Build history of the part. All positions in model axes, mm. A direction names the side the tool comes from. Coordinates: 2 decimals unless noted, no trailing zeros. Loops run counter-clockwise (first coordinate to the right, second up) from the corner with the lowest first, then second, coordinate; pieces in that order, holes last.
Item 1: Drill centre lines: line 1 along X through (y, z) = (11.5, 7); line 2 along Y through (x, z) = (11.5, 6.5); line 3 along X through (y, z) = (10, 8.5). Where is each one in solid material? Low to high.
Item 2: Flat gauge pins, fed straight in: pin 1 (1 mm diameter, centred on x = 0.5, y = 7.5, fed in from -Z); pin 2 (10 mm diameter, centred on x = -11, y = 5, fed in from +Z); pin 3 (4 mm diameter, centred on y = 10, z = -12, fed in from +X). Where does each tip first touch, or does it go through?
Item 3: Cut at C-C (z = 0). List the corners of the cut face in (x, y).
Item 4: Cut at D-D (x = 9.5). List the corners of the cut face in (y, z), and give its area (3 significant figures).
Item 5: Cut at B-B (x = 0). List the corners of the cut face in (y, z) (3 decimals).
Item 6: 3-axis set-ups, long thin cutter, end or side, ignore diameter. For faces 1 (the face through (0, -5, 0.75)), 2 (the face through (-11.03, 7.6, -2.19)), 3 (the face through (2, 15.5, 2)), 4 (the face through (0, -5, -1.5)): which of +Z, -Z, +X, -X, +Y, -Y reach the whole face in a straight line?
Item 7: Mould opens along X. For faces 5 (the face through (5.56, 7.6, 9.91)), 6 (the face through (9.498, 7.395, -12.876)), 7 (the face through (0, 24, -1.25)) say: released by +X, released by -X, zero draft, split by the parting line, or undercut.
from build123d import *

# Parameters (mm, degrees)
SKETCH_1_R               = 16
EXTRUDE_1_DEPTH          = 15
SKETCH_2_R               = 4
EXTRUDE_2_DEPTH          = 0.5
EXTRUDE_START            = 0.5
SKETCH_3_R               = 4
EXTRUDE_3_DEPTH          = 0.5
SKETCH_4_R               = 2.5
EXTRUDE_4_DEPTH          = 9.8
EXTRUDE_START_2          = 3
SKETCH_5_R               = 2.5
EXTRUDE_5_DEPTH          = 3
CUT_EXTRUDE_START        = -2.8
CUT_EXTRUDE_1_DEPTH      = 2.8
CUT_EXTRUDE_2_DEPTH      = 30.227555491
PATTERN_CIRCULAR_1_COUNT = 5
SKETCH_8_R               = 1.5
EXTRUDE_6_DEPTH          = 3
CHAMFER_1_SIZE           = 0.5
CUT_EXTRUDE_START_2      = -3
CUT_EXTRUDE_3_DEPTH      = 3


with BuildPart() as part:
    # 草图1 → 凸台-拉伸1 (new body)
    with BuildSketch(Plane(origin=(0, 0, 0), x_dir=(1, 0, 0), z_dir=(0, 1, 0))):
        with Locations(Location((0, 0, 0), (0, 0, 270))):
            Circle(SKETCH_1_R)
    extrude(amount=EXTRUDE_1_DEPTH)

    # 草图2 → 凸台-拉伸2 (add)
    with BuildSketch(Plane(origin=(0, 15, 0), x_dir=(1, 0, 0), z_dir=(0, 1, 0))):
        with Locations(Location((0, 0, 0), (0, 0, 270))):
            Circle(SKETCH_2_R)
    extrude(amount=EXTRUDE_2_DEPTH)

    # 草图3 → 凸台-拉伸3 (add)
    with BuildSketch(Plane.XZ.offset(EXTRUDE_START)):
        with Locations(Location((0, 0, 0), (0, 0, 90))):
            Circle(SKETCH_3_R)
    extrude(amount=-EXTRUDE_3_DEPTH)

    # 草图4 → 凸台-拉伸4 (add)
    with BuildSketch(Plane(origin=(0, 15.5, 0), x_dir=(1, 0, 0), z_dir=(0, 1, 0))):
        with Locations(Location((0, 0, 0), (0, 0, 270))):
            Circle(SKETCH_4_R)
    extrude(amount=EXTRUDE_4_DEPTH)

    # 草图5 → 凸台-拉伸5 (add)
    with BuildSketch(Plane.XZ.offset(0.5).offset(EXTRUDE_START_2)):
        with Locations(Location((0, 0, 0), (0, 0, 90))):
            Circle(SKETCH_5_R)
    extrude(amount=-EXTRUDE_5_DEPTH)

    # 草图6 → 切除-拉伸1 (cut)
    with BuildSketch(Plane(origin=(0, 25.3, 0), x_dir=(1, 0, 0), z_dir=(0, 1, 0)).offset(CUT_EXTRUDE_START)):
        with BuildLine():
            Line((-2.165063509, 1.25), (2.165063509, 1.25))
            ThreePointArc((2.165063509, 1.25), (0, 2.5), (-2.165063509, 1.25))
        make_face()
    extrude(amount=CUT_EXTRUDE_1_DEPTH, mode=Mode.SUBTRACT)

    # 草图7 → 切除-拉伸2 (cut, through all)
    with BuildSketch(Plane(origin=(0, 15, 0), x_dir=(1, 0, 0), z_dir=(0, 1, 0))):
        with BuildLine():
            Line((-1.325, 7), (-1.325, 19))
            Line((-1.325, 19), (1.325, 19))
            Line((1.325, 19), (1.325, 7))
            ThreePointArc((1.325, 7), (0, 5.675), (-1.325, 7))
        make_face()
    cut_extrude_2 = extrude(amount=-CUT_EXTRUDE_2_DEPTH, mode=Mode.SUBTRACT)

    # 阵列(圆周)1: 切除-拉伸2 ×5 about axis
    pattern_circular_1_axis = Axis((0, 0, 0), (0, 1, 0))
    for i in range(1, PATTERN_CIRCULAR_1_COUNT):
        add(cut_extrude_2.rotate(pattern_circular_1_axis, i * 360 / PATTERN_CIRCULAR_1_COUNT), mode=Mode.SUBTRACT)

    # 草图8 → 凸台-拉伸6 (add)
    with BuildSketch(Plane.XZ.offset(3.5)):
        with Locations(Location((0, 0, 0), (0, 0, 270))):
            Circle(SKETCH_8_R)
    extrude(amount=EXTRUDE_6_DEPTH)

    # 倒角1
    # the kernel refuses this chamfer: 0.5, 0.463229901 mm, written as the material it takes off along each edge
    with BuildSketch(Plane(origin=(-1.325, 16.285841494, -15.945042333), x_dir=(-0.9952786218717831, 0, 0.09705907914772452), z_dir=(0, -1, 0)), Plane(origin=(14.755188896, 16.285841494, -6.187438941), x_dir=(-0.39986667798550435, 0, -0.9165733139453914), z_dir=(0, -1, 0)), Plane(origin=(10.444208248, 16.285841494, 12.120994764), x_dir=(0.7481474239082289, 0, -0.6635325403471037), z_dir=(0, -1, 0)), Plane(origin=(-8.300313213, 16.285841494, 13.678625683), x_dir=(0.8622472145564707, 0, 0.5064876513693177), z_dir=(0, -1, 0)), Plane(origin=(-15.574083931, 16.285841494, -3.667139173), x_dir=(-0.21524933860740833, 0, 0.9765591237754493), z_dir=(0, -1, 0))) as chamfer_1_piece_1:
        with BuildLine():
            Line((0.457733904, 0), (CHAMFER_1_SIZE * 0.0970590791477, -CHAMFER_1_SIZE * 0.995278621872))
            Line((CHAMFER_1_SIZE * 0.0970590791477, -CHAMFER_1_SIZE * 0.995278621872), (0, 0))
            ThreePointArc((0, 0), (0.235215907, 0.001635702), (0.457733904, 0))
        make_face()
    extrude(amount=17.571682988, mode=Mode.SUBTRACT)
    with BuildSketch(Plane(origin=(1.325, 16.285841494, -15.945042333), x_dir=(0, 0, 1), z_dir=(0, -1, 0)), Plane(origin=(15.574083931, 16.285841494, -3.667139173), x_dir=(-0.9510565162951534, 0, 0.3090169943749483), z_dir=(0, -1, 0)), Plane(origin=(8.300313213, 16.285841494, 13.678625683), x_dir=(-0.5877852522924737, 0, -0.809016994374947), z_dir=(0, -1, 0)), Plane(origin=(-14.755188896, 16.285841494, -6.187438941), x_dir=(0.9510565162951536, 0, 0.3090169943749472), z_dir=(0, -1, 0))) as chamfer_1_piece_2:
        with BuildLine():
            Line((CHAMFER_1_SIZE, 0), (0.044427231, -0.455572769))
            ThreePointArc((0.044427231, -0.455572769), (0.02120186, -0.234264124), (0, 0))
            Line((0, 0), (CHAMFER_1_SIZE, 0))
        make_face()
    extrude(amount=17.571682988, mode=Mode.SUBTRACT)
    with BuildSketch(Plane(origin=(-10.444208248, 16.285841494, 12.120994764), x_dir=(-0.7481474239082269, 0, -0.6635325403471058), z_dir=(0, -1, 0))) as chamfer_1_piece_3:
        with BuildLine():
            Line((0.457733904, 0), (CHAMFER_1_SIZE * 0.0970590791477, CHAMFER_1_SIZE * 0.995278621872))
            Line((CHAMFER_1_SIZE * 0.0970590791477, CHAMFER_1_SIZE * 0.995278621872), (0, 0))
            ThreePointArc((0, 0), (0.235215907, -0.001635702), (0.457733904, 0))
        make_face()
    extrude(amount=17.571682988, mode=Mode.SUBTRACT)

    # 草图9 → 切除-拉伸3 (cut)
    with BuildSketch(Plane.XZ.offset(6.5).offset(CUT_EXTRUDE_START_2)):
        with BuildLine():
            Line((-1.299038106, 0.75), (1.299038106, 0.75))
            ThreePointArc((1.299038106, 0.75), (0, 1.5), (-1.299038106, 0.75))
        make_face()
    extrude(amount=CUT_EXTRUDE_3_DEPTH, mode=Mode.SUBTRACT)


solid = part.part
Filled sheet:
1. line 1: x = -14.39 to -6.72, -3.45 to 3.45, 6.72 to 14.39
1. line 2: y = 0 to 15
1. line 3: x = -13.56 to -7.81, -4.54 to 4.54, 7.81 to 13.56
2. pin 1: stops at z = -6.13
2. pin 2: stops at z = 14.83
2. pin 3: stops at x = 12.49
3. outline: (-16, 0) - (-4, 0) - (-4, -0.5) - (-2.5, -0.5) - (-2.5, -3.5) - (-1.5, -3.5) - (-1.5, -6.5) - (1.5, -6.5) - (1.5, -3.5) - (2.5, -3.5) - (2.5, -0.5) - (4, -0.5) - (4, 0) - (16, 0) - (16, 15) - (4, 15) - (4, 15.5) - (2.5, 15.5) - (2.5, 25.3) - (-2.5, 25.3) - (-2.5, 15.5) - (-4, 15.5) - (-4, 15) - (-16, 15) - close
4. outline: (0, -12.87) - (15, -12.87) - (15, -4.48) - (0, -4.48) - close; (0, -1.69) - (15, -1.69) - (15, 10.82) - (0, 10.82) - close
4. area: 314 mm2
5. outline: (-6.5, -1.5) - (-3.5, -1.5) - (-3.5, -2.5) - (-0.5, -2.5) - (-0.5, -4) - (0, -4) - (0, -5.675) - (15, -5.675) - (15, -4) - (15.5, -4) - (15.5, -2.5) - (22.5, -2.5) - (22.5, -1.25) - (25.3, -1.25) - (25.3, 2.5) - (15.5, 2.5) - (15.5, 4) - (15, 4) - (15, 16) - (0, 16) - (0, 4) - (-0.5, 4) - (-0.5, 2.5) - (-3.5, 2.5) - (-3.5, 0.75) - (-6.5, 0.75) - close
6. face 1: +Z, +X, -X, -Y
6. face 2: +Y, -Y
6. face 3: +Y
6. face 4: -Y
7. face 5: undercut
7. face 6: released by +X
7. face 7: zero draft
